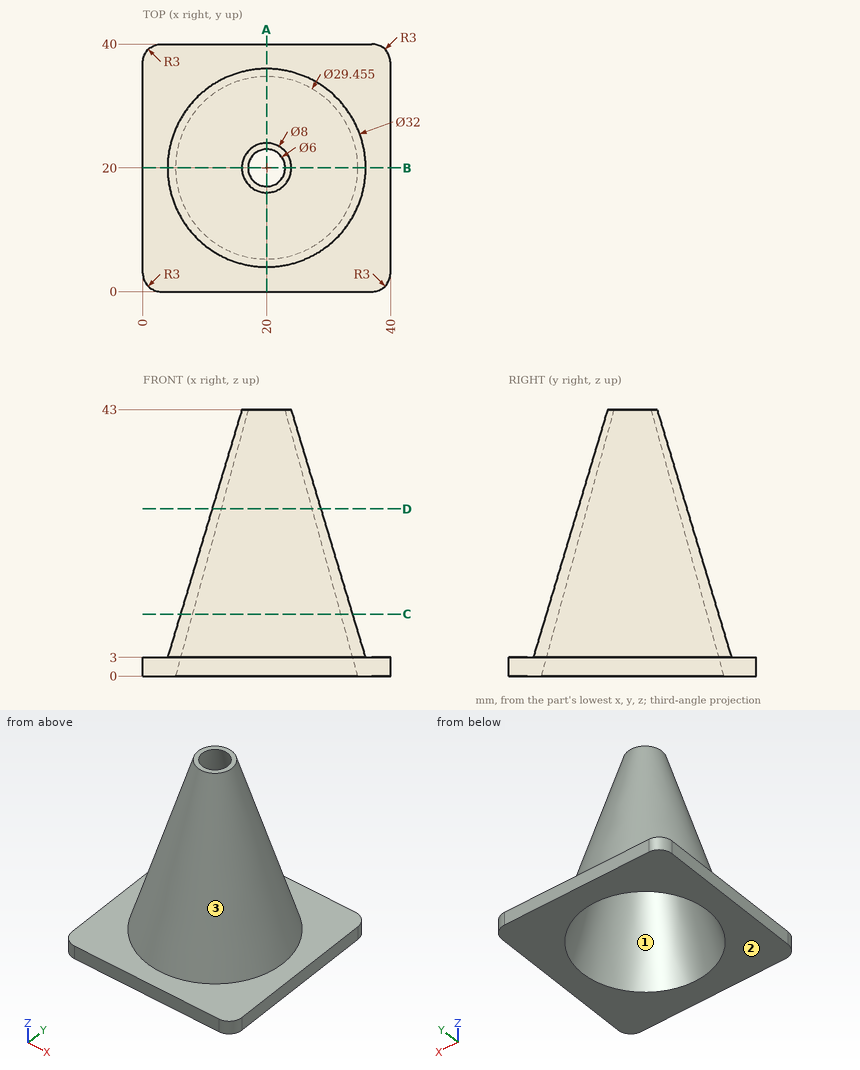
Here's the drawing with two shaded views (mm, measured from the low corner). I have some questions. Coordinates: 2 decimals unless noted, no trailing zeros. Write each loop counter-clockwise with the first axis right and the second up, starting at its lowest first coordinate (ties: lowest second). Pieces come first, ordered by that corner, then holes. Notation, with made-up numbers: M -11.5,-32.75 L 20.5,-32.75 A23 cw 20.5,6.25 Z; hole C 2,14 d10. An arc over 180 degrees is marked long. Answer as CSV lines item,"result". Start each with the question number.
1) Please list where these lines run through material, in increasing order: line 1 (Z direction, x = 21, y = 4); line 2 (Y direction, x = 29, z = 6) (1 decimal); line 3 (X direction, y = 30.5, z = 3.5) (1 decimal). Write a range as from..to.
2) I want a section at A-A, the plane x = 20. Please give me the cut outline in (y, z).
3) We'd pull the mould along X, two halves only. Please class the marked faces 1, 2 and 3: +X half, -X half, draft (parallel to the pull), parting line (faces both ways), or undercut.
4) I want a section at D-D, the plane z = 27. Please give me the cut outline in (x, y).
5) For P1, Ø4, axis at x = 14, z = 31.5, coming from the +Y side; P2, Ø1, axis at x = 18.5, z = 25.5, coming from the +Y side; P3, Ø2, axis at y = 27.5, z = 20, coming from the +X side, each with a flat end and sliding along its axis, tell me the tip position at first contact or that it passes through.
6) I want a section at C-C, the plane z = 10. Please give me the cut outline in (x, y).
Data:
1,line 1,"z = 0..3"
1,line 2,"y = 7.9..10.5, 29.5..32.1"
1,line 3,"x = 8.1..11.1, 28.9..31.9"
2,outline,"M 0,0 L 5.27,0 L 17,43 L 16,43 L 4,3 L 0,3 Z; M 23,43 L 34.73,0 L 40,0 L 40,3 L 36,3 L 24,43 Z"
3,face 1,"undercut"
3,face 2,"draft"
3,face 3,"parting line"
4,outline,"C 20,20 d17.6; hole C 20,20 d14.73"
5,P1,"stops at y = 26.47"
5,P2,"stops at y = 29.3"
5,P3,"stops at x = 28.84"
6,outline,"C 20,20 d27.8; hole C 20,20 d24"
